from build123d import *

# Parameters (mm, degrees)
BOSS_EXTRUDE1_DEPTH = 12.7
SKETCH2_R           = 12.7
BOSS_EXTRUDE2_DEPTH = 25.4
BOSS_EXTRUDE3_START = 12.7
SKETCH3_R           = 12.7
BOSS_EXTRUDE3_DEPTH = 12.7


with BuildPart() as part:
    # Sketch1 → Boss-Extrude1 (new body)
    with BuildSketch(Plane(origin=(0, 0, 0), x_dir=(1, 0, 0), z_dir=(0, 1, 0))):
        with BuildLine():
            ThreePointArc((-50.8, -43.994090512), (-68.148522628, -39.345567884), (-63.5, -21.997045256))
            ThreePointArc((-63.5, -21.997045256), (-26.311818976, 15.191135768), (-12.7, 65.991135768))
            ThreePointArc((-12.7, 65.991135768), (0, 78.691135768), (12.7, 65.991135768))
            ThreePointArc((12.7, 65.991135768), (26.311818976, 15.191135768), (63.5, -21.997045256))
            ThreePointArc((63.5, -21.997045256), (68.148522628, -39.345567884), (50.8, -43.994090512))
            ThreePointArc((50.8, -43.994090512), (0, -30.382271537), (-50.8, -43.994090512))
        make_face()
    extrude(amount=BOSS_EXTRUDE1_DEPTH)

    # Sketch2 → Boss-Extrude2 (add)
    with BuildSketch(Plane(origin=(0, 12.7, 0), x_dir=(1, 0, 0), z_dir=(0, 1, 0))):
        with Locations(Location((0, 0, 0), (0, 0, 270))):
            Circle(SKETCH2_R)
    extrude(amount=BOSS_EXTRUDE2_DEPTH)

    # Sketch3 → Boss-Extrude3 (add)
    with BuildSketch(Plane.XZ.offset(BOSS_EXTRUDE3_START)):
        with Locations(Location((-57.15, 32.995567884, 0), (0, 0, 270))):
            Circle(SKETCH3_R)
        with Locations(Location((57.15, 32.995567884, 0), (0, 0, 270))):
            Circle(SKETCH3_R)
        with Locations(Location((0, -65.991135768, 0), (0, 0, 270))):
            Circle(SKETCH3_R)
    extrude(amount=-BOSS_EXTRUDE3_DEPTH)


solid = part.part
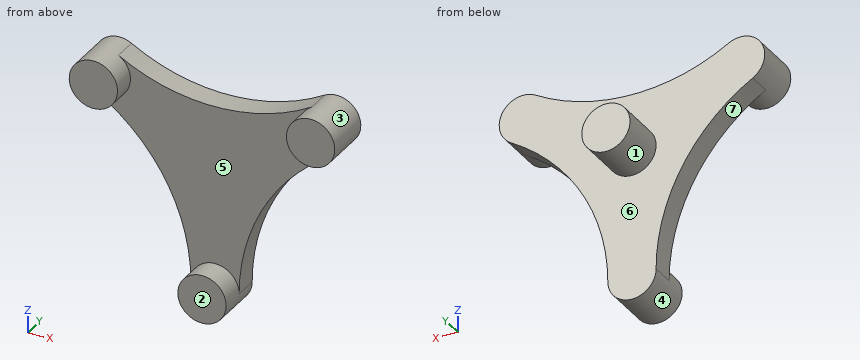
The model under review builds one solid part; all positions refer to its coordinate system, in mm. Face numbers are marked on the shaded views. A direction names the side the tool comes from. Coordinates: 2 decimals unless noted, no trailing zeros. Write each loop counter-clockwise with the first axis right and the second up, starting at its lowest first coordinate (ties: lowest second). Pieces come first, ordered by that corner, then holes. Notation, with made-up numbers: (51, 57.25) -> (103, 57.25) arc R25 ccw to (103, 73.25) -> close; hole circle Ø7 at (13, 2.5). An arc over 180 degrees is marked (long way). Answer in a Markdown table with one row per item.
1. We need section C-C, the plane z = 0. State the section outline as (x, y) points.
Answers below:
| item | result |
|---|---|
| outline | (-37.05, 0) -> (37.05, 0) -> (37.05, 12.7) -> (12.7, 12.7) -> (12.7, 38.1) -> (-12.7, 38.1) -> (-12.7, 12.7) -> (-37.05, 12.7) -> close |
2. Draft analysis for pull direction X (two halves, no side actions). For the marked faces 4, 5, 6 and 7, state which applies: +X half, -X half, draft (parallel to the pull), parting line (faces both ways), or undercut.
Answers below:
| item | result |
|---|---|
| face 4 | parting line |
| face 5 | undercut |
| face 6 | draft |
| face 7 | -X half |
3. We need section B-B, the plane y = 11. State the section outline as (x, z) points.
Answers below:
| item | result |
|---|---|
| outline | (-63.5, 22) arc R101.6 cw to (-12.7, -65.99) arc R12.7 ccw to (12.7, -65.99) arc R101.6 cw to (63.5, 22) arc R12.7 ccw to (50.8, 43.99) arc R101.6 cw to (-50.8, 43.99) arc R12.7 ccw to start |
4. We need section A-A, the plane z = 33.5. State the section outline as (x, y) points.
Answers below:
| item | result |
|---|---|
| outline | (-69.84, -12.7) -> (-44.46, -12.7) -> (-44.46, 0) -> (-24.98, 0) -> (-24.98, 12.7) -> (-69.84, 12.7) -> close; (24.98, 0) -> (44.46, 0) -> (44.46, -12.7) -> (69.84, -12.7) -> (69.84, 12.7) -> (24.98, 12.7) -> close |
5. Wall thickness on probe 1 along Y at (x, z) = (-10, -34); probe 2 along Z at (x, y) = (0.5, 17); probe 3 along X at (y, z) = (-8.5, 35.5): over which ranges is each line inside the solid? List them lowest first. Write a range as [from, to].
Answers below:
| item | result |
|---|---|
| probe 1 | y = [0, 12.7] |
| probe 2 | z = [-12.69, 12.69] |
| probe 3 | x = [-69.6, -44.7], [44.7, 69.6] |
6. For the marked faces 1, 2 and 3, list the 3-axis set-ups (+Z, -Z, +X, -X, +Y, -Y) from which the entire face can be reached by the end or side of a thin tool; tool diameter is ignored.
Answers below:
| item | result |
|---|---|
| face 1 | +Y |
| face 2 | +Z, -Z, +X, -X, -Y |
| face 3 | -Y |
7. We need section D-D, the plane x = 57.15. State the section outline as (y, z) points, and give its area (3 significant figures).
Answers below:
| item | result |
|---|---|
| outline | (-12.7, 20.3) -> (0, 20.3) -> (0, 18.01) -> (12.7, 18.01) -> (12.7, 45.7) -> (-12.7, 45.7) -> close |
| area | 674 mm^2 |
8. Clearance check with flat-ended pins moving along their axes: pin 1 Ø5 at (x, y) = (44, 13.5) entering from +Z; pin 2 Ø5 at (y, z) = (8, 4) entering from -X; pin 3 Ø5 at (y, z) = (-3, 10) entering from -X; pin 4 Ø3 at (y, z) = (12.5, -30) entering from +X. State where each tip first meets the part, or that it passes through.
Answers below:
| item | result |
|---|---|
| pin 1 | stops at z = 41.58 |
| pin 2 | stops at x = -43.11 |
| pin 3 | passes through |
| pin 4 | stops at x = 19.87 |
